from build123d import *

# Parameters (mm, degrees)
SKETCH_1_R      = 1.5
SKETCH_1_R_2    = 4.5
SKETCH_1_R_3    = 3.5
EXTRUDE_1_DEPTH = 1.5


with BuildPart() as part:
    # 草图1 → 凸台-拉伸1 (new body)
    with BuildSketch(Plane.XY):
        with BuildLine():
            Line((-14.119787017, 9.298767484), (-75.323772101, 5.991257934))
            ThreePointArc((-75.323772101, 5.991257934), (-81, 0), (-75.323772101, -5.991257934))
            Line((-75.323772101, -5.991257934), (-14.119787017, -9.298767484))
            ThreePointArc((-14.119787017, -9.298767484), (-10.458227409, -9.958733326), (-7.071734496, -11.499590046))
            ThreePointArc((-7.071734496, -11.499590046), (13.5, 0), (-7.071734496, 11.499590046))
            ThreePointArc((-7.071734496, 11.499590046), (-10.458227409, 9.958733326), (-14.119787017, 9.298767484))
        make_face()
        with Locations((-5.656854249, -5.656854249)):
            Circle(SKETCH_1_R, mode=Mode.SUBTRACT)
        with Locations((-6.717514421, 6.717514421)):
            Circle(SKETCH_1_R, mode=Mode.SUBTRACT)
        with Locations((5.656854249, 5.656854249)):
            Circle(SKETCH_1_R, mode=Mode.SUBTRACT)
        with Locations((6.717514421, -6.717514421)):
            Circle(SKETCH_1_R, mode=Mode.SUBTRACT)
        Circle(SKETCH_1_R_2, mode=Mode.SUBTRACT)
        with Locations((-60, 0)):
            Circle(SKETCH_1_R_3, mode=Mode.SUBTRACT)
        with Locations((-75, 0)):
            Circle(SKETCH_1_R_3, mode=Mode.SUBTRACT)
        with BuildLine():
            Line((-19.5, 5.475889357), (-19.5, -5.137613899))
            ThreePointArc((-19.5, -5.137613899), (-19.75, -5.570626601), (-20.25, -5.570626601))
            Line((-20.25, -5.570626601), (-37.059715141, 4.134466961))
            ThreePointArc((-37.059715141, 4.134466961), (-37.295994973, 4.683806463), (-36.836696149, 5.066751157))
            Line((-36.836696149, 5.066751157), (-20.026981008, 5.975160851))
            ThreePointArc((-20.026981008, 5.975160851), (-19.656118119, 5.838856645), (-19.5, 5.475889357))
        make_face(mode=Mode.SUBTRACT)
        with BuildLine():
            Line((-43.593398767, 4.442589346), (-27.929722665, -4.600838268))
            ThreePointArc((-27.929722665, -4.600838268), (-27.700428576, -5.176248922), (-28.206703673, -5.533122464))
            Line((-28.206703673, -5.533122464), (-49.030790414, -4.407773099))
            ThreePointArc((-49.030790414, -4.407773099), (-49.449681707, -4.134771113), (-49.422700699, -3.635499618))
            Line((-49.422700699, -3.635499618), (-44.262290061, 4.28257863))
            ThreePointArc((-44.262290061, 4.28257863), (-43.959725568, 4.495856477), (-43.593398767, 4.442589346))
        make_face(mode=Mode.SUBTRACT)
    extrude(amount=EXTRUDE_1_DEPTH)


solid = part.part
Part model, mm, in its own coordinate system. A direction names the side the tool comes from. Coordinates: 2 decimals unless noted, no trailing zeros. Order: outer loops, then holes, each group sorted by start corner. A loop starts at its lowest first (then second) coordinate and runs counter-clockwise, first axis right, second up. Notation, with made-up numbers: M 1.5,61 L 49.5,61 A26 ccw 49.5,94 Z; hole C 42,74.5 d6. An arc over 180 degrees is marked long. One line per question, with ' | ' between items.
Q1. Drill centre lines: line 1 (X direction, y = -0.5, z = 0.6); line 2 (X direction, y = -3.75, z = 0.25); line 3 (Y direction, x = -7, z = 0.6). Where is each one in solid material? Low to high.
A:
line 1: x = -80.98 to -78.46, -71.54 to -63.46, -56.54 to -47.38, -35.03 to -29.03, -19.5 to -4.47, 4.47 to 13.49 | line 2: x = -79.68 to -49.48, -29.4 to -23.4, -19.5 to -2.49, 2.49 to 12.97 | line 3: y = -11.54 to -6.32, -4.99 to 5.24, 8.19 to 11.54
Q2. Slice it at C-C (z = 0.35). Count the separate pieces of the cut face and the enclosed holes in it, and give its area (3 significant figures).
A:
separate pieces: 1 | enclosed holes: 9 | area: 1,210 mm^2
Q3. Pin check, flat tip, straight feed: P1, Ø8, axis at x = 0, y = 0, coming from the -Z side. Stop position of the tip, or through.
A:
P1: passes through
Q4. Slice it at B-B (y = 0). Give the cut face in (x, z).
A:
outline: M -81,0 L -78.5,0 L -78.5,1.5 L -81,1.5 Z; M -71.5,0 L -63.5,0 L -63.5,1.5 L -71.5,1.5 Z; M -56.5,0 L -47.05,0 L -47.05,1.5 L -56.5,1.5 Z; M -35.9,0 L -29.9,0 L -29.9,1.5 L -35.9,1.5 Z; M -19.5,0 L -4.5,0 L -4.5,1.5 L -19.5,1.5 Z; M 4.5,0 L 13.5,0 L 13.5,1.5 L 4.5,1.5 Z
Q5. Slice it at D-D (x = -41.5). Give the cut face in (y, z), and give its area (3 significant figures).
A:
outline: M -7.82,0 L -4.81,0 L -4.81,1.5 L -7.82,1.5 Z; M 3.23,0 L 7.82,0 L 7.82,1.5 L 3.23,1.5 Z | area: 11.4 mm^2
Q6. Two-plate mould, pull along Y, no slides. Class faces 3 (the face through (-24, 6, 1.5)), 4 (the face through (-45.15, -7.62, 0.74)), 5 (the face through (-35.9, 0, 0.7)), 6 (the face through (-0.59, 4.46, 0.74)): +Y half, -Y half, draft (parallel to the pull), parting line (faces both ways), or undercut.
A:
face 3: draft | face 4: -Y half | face 5: undercut | face 6: undercut
Q7. 3-axis set-ups, long thin cutter, end or side, ignore diameter. For faces 1 (the face through (-38.47, -4.98, 0.74)), 2 (the face through (-10.408, 9.974, 0.74)): which of +Z, -Z, +X, -X, +Y, -Y reach the whole face in a straight line?
A:
face 1: +Z, -Z | face 2: +Z, -Z, -X, +Y
Q8. Slice it at A-A (x = 0). Give the cut face in (y, z), and give its area (3 significant figures).
A:
outline: M -13.5,0 L -4.5,0 L -4.5,1.5 L -13.5,1.5 Z; M 4.5,0 L 13.5,0 L 13.5,1.5 L 4.5,1.5 Z | area: 27.0 mm^2
